from build123d import *

# Parameters (mm, degrees)
BOSS_EXTRUDE1_DEPTH                              = 330.0000000000001
CUT_EXTRUDE1_DEPTH                               = 331.15148038439605
CUT_EXTRUDE2_DEPTH                               = 331.15148038439605
CUT_EXTRUDE3_DEPTH                               = 331.15148038439605
CUT_EXTRUDE4_DEPTH                               = 331.15148038439605
CUT_EXTRUDE5_DEPTH                               = 331.15148038439605
CBORE_FOR_M3_HEX_HEAD_MACHINE_SCREW1_D           = 3.5
CBORE_FOR_M3_HEX_HEAD_MACHINE_SCREW1_CBORE_D     = 6
CBORE_FOR_M3_HEX_HEAD_MACHINE_SCREW1_CBORE_DEPTH = 4.500000001
CHAMFER1_SIZE                                    = 0.49999999999999817
FILLET1_R                                        = 0.2499999999999934


with BuildPart() as part:
    # Sketch1 → Boss-Extrude1 (new body)
    with BuildSketch(Plane(origin=(315, 0, 0), x_dir=(0, 0, -1), z_dir=(1, 0, 0))):
        Polygon((-6.645656211367382, -5.999999999987301), (-6.086528667804737, -5.9999999999873), (-4.3218662036368185, -5.999999999987301), (-4.142120421, -5.999999999987301), (-0.5, -5.999999999987301), (1.1e-16, -5.999999999987301), (1.1e-16, -5.499999999987301), (1.1e-16, 1.6000000000126995), (1.1e-16, 2.4000000000130934), (1.1e-16, 5.500000000038499), (1.1e-16, 6.000000000012701), (-0.5, 6.000000000012701), (-4.142120421, 6.000000000012701), (-4.321866203637508, 6.000000000012701), (-6.086528667804739, 6.000000000012701), (-6.645656211361536, 6.000000000012701), (-6.8254019940016, 6.0000000000127), (-7.5000000005016, 6.0000000000127), (-8.0000000005016, 5.500000000012699), (-8.0000000005016, -5.4999999999873), (-7.5000000005016, -5.9999999999873), (-6.8254019940016, -5.9999999999873), align=None)
    extrude(amount=-BOSS_EXTRUDE1_DEPTH)

    # Sketch2 → Cut-Extrude1 (cut, through all)
    with BuildSketch(Plane.ZY.offset(15.000000000000124)):
        with BuildLine():
            Line((6.08652866780937, -6.000000000000199), (6.018802044260312, -5.225881150429053))
            Line((6.018802044260312, -5.225881150429053), (6.00733187975836, -5.094776570230831))
            Line((6.00733187975836, -5.094776570230831), (5.975261553557278, -4.728211064330927))
            Line((5.975261553557278, -4.728211064330927), (5.955295672541693, -4.500000000017885))
            Line((5.955295672541693, -4.500000000017885), (5.726212879033703, -4.500000000017885))
            Line((5.726212879033703, -4.500000000017885), (5.273791122033704, -4.500000000017885))
            Line((5.273791122033704, -4.500000000017885), (5.044708328549826, -4.500000000017885))
            Line((5.044708328549826, -4.500000000017885), (5.024742447510704, -4.728211064330986))
            Line((5.024742447510704, -4.728211064330986), (4.994504855310705, -5.073828324330986))
            Line((4.994504855310705, -5.073828324330986), (4.982621846705465, -5.209651734063311))
            ThreePointArc((4.982621846705465, -5.209651734063311), (4.5631182691832715, -5.530313973033924), (4.321866203641435, -6.000000000000199))
            Line((4.321866203641435, -6.000000000000199), (6.08652866780937, -6.000000000000199))
        make_face()
    extrude(amount=-CUT_EXTRUDE1_DEPTH, mode=Mode.SUBTRACT)

    # Sketch3 → Cut-Extrude2 (cut, through all)
    with BuildSketch(Plane.ZY.offset(15.000000000000124)):
        with BuildLine():
            Line((4.63134e-12, 2.4000000000000923), (4.63324e-12, 1.5999999999997847))
            ThreePointArc((4.63324e-12, 1.5999999999997847), (0.20000000000487567, 1.9999999999999392), (4.63134e-12, 2.4000000000000923))
        make_face()
    extrude(amount=-CUT_EXTRUDE2_DEPTH, mode=Mode.SUBTRACT)

    # Sketch4 → Cut-Extrude3 (cut, through all)
    with BuildSketch(Plane.ZY.offset(15.000000000000124)):
        with BuildLine():
            Line((6.007331879761033, 5.0947765702430985), (6.018802044262717, 5.225881150442735))
            Line((6.018802044262717, 5.225881150442735), (6.08652866780937, 6.0000000000127))
            Line((6.08652866780937, 6.0000000000127), (4.3218662036421405, 6.0000000000127))
            ThreePointArc((4.3218662036421405, 6.0000000000127), (4.563118269185973, 5.530313973045934), (4.982621846709898, 5.209651734075363))
            Line((4.982621846709898, 5.209651734075363), (4.994504855315133, 5.0738283243431))
            Line((4.994504855315133, 5.0738283243431), (5.024742447515134, 4.728211064343101))
            Line((5.024742447515134, 4.728211064343101), (5.044708328554257, 4.50000000003))
            Line((5.044708328554257, 4.50000000003), (5.273791122038133, 4.50000000003))
            Line((5.273791122038133, 4.50000000003), (5.7262128790381315, 4.50000000003))
            Line((5.7262128790381315, 4.50000000003), (5.9552956725461215, 4.50000000003))
            Line((5.9552956725461215, 4.50000000003), (5.975261553561033, 4.728211064343099))
            Line((5.975261553561033, 4.728211064343099), (6.007331879761033, 5.0947765702430985))
        make_face()
    extrude(amount=-CUT_EXTRUDE3_DEPTH, mode=Mode.SUBTRACT)

    # Sketch5 → Cut-Extrude4 (cut, through all)
    with BuildSketch(Plane.ZY.offset(15.000000000000124)):
        with BuildLine():
            Line((6.086528667809372, 6.0000000000127), (6.018802044262717, 5.225881150442735))
            ThreePointArc((6.018802044262717, 5.225881150442735), (6.4163451501653705, 5.544826384286438), (6.645656211366141, 6.0000000000127))
            Line((6.645656211366141, 6.0000000000127), (6.086528667809372, 6.0000000000127))
        make_face()
    extrude(amount=-CUT_EXTRUDE4_DEPTH, mode=Mode.SUBTRACT)

    # Sketch6 → Cut-Extrude5 (cut, through all)
    with BuildSketch(Plane.ZY.offset(15.000000000000124)):
        with BuildLine():
            Line((6.08652866780937, -5.999999999987301), (6.645656211368704, -5.999999999987301))
            ThreePointArc((6.645656211368704, -5.999999999987301), (6.416345150166451, -5.544826384259201), (6.018802044260312, -5.225881150416156))
            Line((6.018802044260312, -5.225881150416156), (6.08652866780937, -5.999999999987301))
        make_face()
    extrude(amount=-CUT_EXTRUDE5_DEPTH, mode=Mode.SUBTRACT)

    # CBORE for M3 Hex Head Machine Screw1 (through all)
    with Locations(Plane.XY.offset(8.0000000005016)):
        with Locations((300, 0), (25, 0), (50, 0), (75, 0), (100, 0), (125, 0), (150, 0), (175, 0), (200, 0), (225, 0), (250, 0), (275, 0), (0, 0)):
            CounterBoreHole(CBORE_FOR_M3_HEX_HEAD_MACHINE_SCREW1_D / 2, CBORE_FOR_M3_HEX_HEAD_MACHINE_SCREW1_CBORE_D / 2, CBORE_FOR_M3_HEX_HEAD_MACHINE_SCREW1_CBORE_DEPTH)

    # Chamfer1
    chamfer1_edges = [part.edges().sort_by_distance(p)[0] for p in [
        (149.99999999999994, 6.000000000012701, -1.1e-16),
        (149.99999999999994, -5.999999999987301, -1.1e-16),
    ]]
    chamfer(chamfer1_edges, length=CHAMFER1_SIZE)

    # Fillet1
    fillet1_edges = [part.edges().sort_by_distance(p)[0] for p in [
        (149.99999999999994, 4.50000000003, 5.955295672546116),
        (149.99999999999994, 4.50000000003, 5.044708328554251),
        (149.99999999999994, 5.209651734075363, 4.982621846709892),
        (149.99999999999994, 6.0000000000127, 4.321866203642135),
        (149.99999999999994, 6.0000000000127, 6.645656211366136),
        (149.99999999999994, 5.225881150442735, 6.018802044262712),
        (149.99999999999994, -5.225881150416156, 6.0188020442603065),
        (149.99999999999994, -5.999999999987301, 6.645656211368698),
        (149.99999999999994, -6.000000000000199, 4.32186620364143),
        (149.99999999999994, -5.209651734063311, 4.9826218467054595),
        (149.99999999999994, -4.500000000017885, 5.044708328549821),
        (149.99999999999994, -4.500000000017885, 5.955295672541688),
    ]]
    fillet(fillet1_edges, radius=FILLET1_R)


solid = part.part
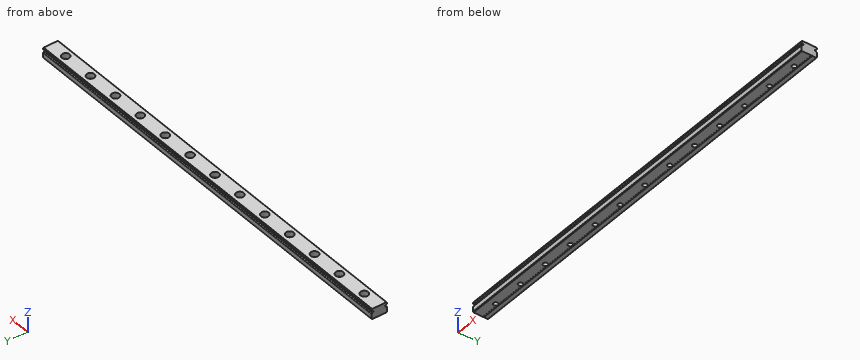
Can you work these out from the model? Positions are in its coordinate system, mm. Coordinates: 2 decimals unless noted, no trailing zeros. Write each question's results on one line, items separated by ' | '. Start each with the question number.
Q1. I'm going to push a flat-ended pin straight in: pin 1 (5.5 mm diameter, centred on x = 175, y = 0, fed in from +Z). Where does the tip first touch, or does it pass through?
Q2. Imagine slicing it at A-A (z = 2). State how many separate pieces and enclosed holes the cut face has, then the cut area to 3 significant figures.
Q3. If I drill on probe 1 along Y at (x, z) = (125, 4.4); probe 2 along Y at (x, z) = (125, 1.6); probe 3 along Y at (x, z) = (37.5, 4.25), over which ranges is the centre line in solid material (lowest first)?
Taken from the geometry:
1) pin 1: stops at z = 3.5
2) separate pieces: 1 | enclosed holes: 13 | area: 3,830 mm^2
3) probe 1: y = -5.78 to -3, 3 to 5.78 | probe 2: y = -6 to -1.75, 1.75 to 6 | probe 3: y = -5.98 to 5.98
